For this review, take the finished solid that the model builds, in its own axes (mm). Face numbers are marked on the shaded views. A direction names the side the tool comes from. Give positions to 0.01 mm unless a question says otherwise; leave off trailing zeros. Order: outer loops, then holes, each group sorted by start corner. A loop starts at its lowest first (then second) coordinate and runs counter-clockwise, first axis right, second up. Notation, with made-up numbers: M 88.5,63 L 129.5,63 A8 cw 129.5,73 Z; hole C -14.75,42 d10. An arc over 180 degrees is marked long. Answer as CSV lines item,"result". Start each with the question number.
1. For line 1 along Y through (x, z) = (9.5, -0.9); line 2 along Y through (x, z) = (-9.5, -0.75); line 3 along Y through (x, z) = (-2.25, -5.5), list the stretches that pass through material, from the lowest coordinate up.
2. We need section C-C, the plane x = 0. Give the boundary of the cut face in (y, z).
3. Machinability: for the marked faces 1, 2 and 3, which of the approach directions +Z, -Z, +X, -X, +Y, -Y give a long, thin tool a straight path to every point of the face, cutting with its end or side? Answer none if there is none.
4. Clearance check with flat-ended pins moving along their axes: P1, Ø5.5, axis at x = 1, z = -15, coming from the +Y side; P2, Ø3.5, axis at y = 2.5, z = -10.5, coming from the -X side; P3, Ø9.5, axis at y = 2.5, z = -20, coming from the +X side. State where each tip first meets the part, or that it passes through.
5. We need section B-B, the plane z = -13.5. Give the boundary of the cut face in (x, y), and give its area (3 significant figures).
6. We need section A-A, the plane y = 0. Give the boundary of the cut face in (x, z).
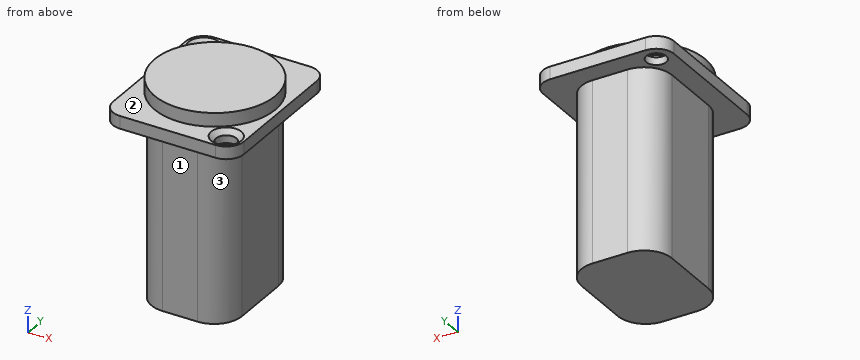
from build123d import *

# Parameters (mm, degrees)
SKETCH1_R           = 2
BOSS_EXTRUDE1_DEPTH = 1.25
BOSS_EXTRUDE2_START = 1.25
SKETCH1_3_R         = 12
BOSS_EXTRUDE2_DEPTH = 2.7
BOSS_EXTRUDE3_START = -1.25
BOSS_EXTRUDE3_DEPTH = 36
CHAMFER1_SIZE       = 1


with BuildPart() as part:
    # Sketch1 → Boss-Extrude1 (new, symmetric)
    with BuildSketch(Plane.XY):
        with BuildLine():
            Line((-9.5, -15.5), (9.5, -15.5))
            ThreePointArc((9.5, -15.5), (11.974873734, -14.474873734), (13, -12))
            Line((13, -12), (13, 12))
            ThreePointArc((13, 12), (11.974873734, 14.474873734), (9.5, 15.5))
            Line((9.5, 15.5), (-9.5, 15.5))
            ThreePointArc((-9.5, 15.5), (-11.974873734, 14.474873734), (-13, 12))
            Line((-13, 12), (-13, -12))
            ThreePointArc((-13, -12), (-11.974873734, -14.474873734), (-9.5, -15.5))
        make_face()
        with Locations((-9.5, 12)):
            Circle(SKETCH1_R, mode=Mode.SUBTRACT)
        with Locations((9.5, -12)):
            Circle(SKETCH1_R, mode=Mode.SUBTRACT)
    extrude(amount=BOSS_EXTRUDE1_DEPTH, both=True)

    # Sketch1<3> → Boss-Extrude2 (add)
    with BuildSketch(Plane.XY.offset(BOSS_EXTRUDE2_START)):
        with Locations(Location((0, 0, 0), (0, 0, 180))):
            Circle(SKETCH1_3_R)
    extrude(amount=BOSS_EXTRUDE2_DEPTH)

    # Sketch1<4> → Boss-Extrude3 (add)
    with BuildSketch(Plane.XY.offset(BOSS_EXTRUDE3_START)):
        with BuildLine():
            Line((-3.464466094, -11.5), (3.464466094, -11.5))
            ThreePointArc((3.464466094, -11.5), (7.378679656, -9.878679656), (9, -5.964466094))
            Line((9, -5.964466094), (9, 5.964466094))
            ThreePointArc((9, 5.964466094), (7.378679656, 9.878679656), (3.464466094, 11.5))
            Line((3.464466094, 11.5), (-3.464466094, 11.5))
            ThreePointArc((-3.464466094, 11.5), (-7.378679656, 9.878679656), (-9, 5.964466094))
            Line((-9, 5.964466094), (-9, -5.964466094))
            ThreePointArc((-9, -5.964466094), (-7.378679656, -9.878679656), (-3.464466094, -11.5))
        make_face()
    extrude(amount=-BOSS_EXTRUDE3_DEPTH)

    # Chamfer1
    chamfer1_edges = [part.edges().sort_by_distance(p)[0] for p in [
        (7.5, -12, 1.25),
        (-11.5, 12, 1.25),
    ]]
    chamfer(chamfer1_edges, length=CHAMFER1_SIZE)


solid = part.part
Result set:
1,line 1,"-15.5 to -14, -10 to 15.5"
1,line 2,"-15.5 to 10, 14 to 15.5"
1,line 3,"-11.5 to 11.5"
2,outline,"M -15.5,-1.25 L -11.5,-1.25 L -11.5,-37.25 L 11.5,-37.25 L 11.5,-1.25 L 15.5,-1.25 L 15.5,1.25 L 12,1.25 L 12,3.95 L -12,3.95 L -12,1.25 L -15.5,1.25 Z"
3,face 1,"-Z, +X, -X, -Y"
3,face 2,"+Z"
3,face 3,"-Z, +X, -Y"
4,P1,"y = 11.5"
4,P2,"x = -9"
4,P3,"x = 9"
5,outline,"M -9,-5.96 A5.54 ccw -3.46,-11.5 L 3.46,-11.5 A5.54 ccw 9,-5.96 L 9,5.96 A5.54 ccw 3.46,11.5 L -3.46,11.5 A5.54 ccw -9,5.96 Z"
5,area,"388 mm2"
6,outline,"M -13,-1.25 L -9,-1.25 L -9,-37.25 L 9,-37.25 L 9,-1.25 L 13,-1.25 L 13,1.25 L 12,1.25 L 12,3.95 L -12,3.95 L -12,1.25 L -13,1.25 Z"
